Could you check a few things on this model? Use its own coordinates, in mm. A direction names the side the tool comes from. Give positions to 0.01 mm unless a question says otherwise; leave off trailing zeros. Loops run counter-clockwise (first coordinate to the right, second up) from the corner with the lowest first, then second, coordinate; pieces in that order, holes last. Notation, with made-up numbers: M -20,43 L 21,43 A26 ccw 21,75 Z; hole C -12,-17 d7. An arc over 180 degrees is marked long. Return JSON: item names as keys, results as strings. Group by question number.
1. If we section it at A-A (y = -23): Write out the boundary of the cut face in (x, z), plus the area to 3 significant figures.
2. Please list where these lines run through material, in increasing order: line 1 (Y direction, x = -20.5, z = 41); line 2 (X direction, y = -4, z = 31.5); line 3 (X direction, y = -6, z = 130).
3. If we section it at C-C (x = 125.5): Write out the boundary of the cut face in (y, z).
4. If we mould it in two halves opening along Z, with no side actions, what happens to faces 4 (the cylindrical face through (86.45, -3.13, 20.73)), 5 (the flat face through (41, -6.35, 53)), 6 (the cylindrical face through (-39.79, -3.22, 1.59))? For each: +Z half, -Z half, draft (parallel to the pull), parting line (faces both ways), or undercut.
5. For faces 1 (the flat face through (162.27, -18.87, 120.88)), 2 (the cylindrical face through (39.885, -3.219, 1.509)), 3 (the flat face through (41, 0, 53)), which set-ups out of +Z, -Z, +X, -X, +Y, -Y let a thin tool reach every point of the face, with its end or its side?
6. If we section it at B-B (z = 80): Write out the boundary of the cut face in (x, y), plus the area to 3 significant figures.
7. For pin 1 (8 mm diameter, centred on y = -15.5, z = 98, fed in from -X); pin 2 (12 mm diameter, centred on x = -55.99, z = 55.99, fed in from -Y); pin 3 (8 mm diameter, centred on x = 127.5, y = -13.5, fed in from +Z), each with a flat end and sliding along its axis, tell me the tip position at first contact or that it passes through.
8. If we section it at D-D (y = -9.5): Write out the boundary of the cut face in (x, z), plus the area to 3 significant figures.
```python
from build123d import *

# Parameters (mm, degrees)
F1_DEPTH = 6.35
F3_D     = 10.3124
F5_DEPTH = 25.4
F7_D     = 14
F8_R     = 12.7
F9_R     = 5.08
F10_R    = 6.35


# Not quite as in the source:
# - a feature names something its author has since deleted; it is built from what else it names


with BuildPart() as f1:
    # F0 (on Front) → F1 (new body)
    with BuildSketch(Plane.XZ):
        with BuildLine():
            Line((38.1, 0), (88.9, 0))
            ThreePointArc((88.9, 0), (85.8708059571, 23.0090131096), (76.9896583964, 44.45))
            Line((76.9896583964, 44.45), (179.5459910838, 103.6609262841))
            Line((179.5459910838, 103.6609262841), (160.4959910838, 136.6564941683))
            Line((160.4959910838, 136.6564941683), (50.5107648032, 73.1564941683))
            ThreePointArc((50.5107648032, 73.1564941683), (-41.3086129578, 78.7198100576), (-88.9, 0))
            Line((-88.9, 0), (-38.1, 0))
            ThreePointArc((-38.1, 0), (0, 38.1), (38.1, 0))
        make_face()
    extrude(amount=F1_DEPTH)

    # F3 (through all)
    with Locations(Plane.XZ.offset(6.35)):
        with Locations((-55.9918969149, 55.9918969149), (55.9918969149, 55.9918969149)):
            Hole(F3_D / 2)

    # F4 (on face) → F5 (join)
    with BuildSketch(Plane.XZ.offset(6.35)):
        Polygon((160.4959910838, 136.6564941683), (154.9967297697, 133.4814941683), (174.0467297697, 100.4859262841), (179.5459910838, 103.6609262841), align=None)
    extrude(amount=F5_DEPTH)

    # F7 (through all)
    with Locations(Plane(origin=(174.0467297697, 0, 100.4859262841), x_dir=(0, -1, 0), z_dir=(-0.8660254038, 0, -0.5))):
        with Locations((19.05, 12.7)):
            Hole(F7_D / 2)

    # F8
    f8_edges = [f1.edges().sort_by_distance(p)[0] for p in [
        (50.510765, -3.175, 73.156494),
        (76.989658, -3.175, 44.45),
    ]]
    fillet(f8_edges, radius=F8_R)

    # F9
    f9_edges = [f1.edges().sort_by_distance(p)[0] for p in [
        (170.020991, 0, 120.15871),
    ]]
    fillet(f9_edges, radius=F9_R)

    # F10
    f10_edges = [f1.edges().sort_by_distance(p)[0] for p in [
        (88.9, -3.175, 0),
        (38.1, -3.175, 0),
        (-38.1, -3.175, 0),
        (-88.9, -3.175, 0),
    ]]
    fillet(f10_edges, radius=F10_R)


solid = f1.part
```
Answer:
{
 "1": {"outline": "M 155,133.48 L 164.81,116.49 L 170.31,119.66 L 160.5,136.66 Z; M 170.59,106.48 L 174.05,100.49 L 179.55,103.66 L 176.09,109.65 Z", "area": "169 mm²"},
 "2": {"line 1": "y = -6.35 to 0", "line 2": "x = -83.13 to -21.43, 21.43 to 83.13", "line 3": "x = 148.97 to 164.34"},
 "3": {"outline": "M -6.35,72.46 L 0,72.46 L 0,116.45 L -6.35,116.45 Z"},
 "4": {"face 4": "undercut", "face 5": "draft", "face 6": "-Z half"},
 "5": {"face 1": "-Z, -X, -Y", "face 2": "-Z, +Y, -Y", "face 3": "+Z, -Z, +X, -X, +Y"},
 "6": {"outline": "M -38.77,-6.35 L 38.77,-6.35 L 38.77,0 L -38.77,0 Z; M 62.36,-6.35 L 138.56,-6.35 L 138.56,0 L 62.36,0 Z", "area": "976 mm²"},
 "7": {"pin 1": "stops at x = 173.17", "pin 2": "stops at y = -6.35", "pin 3": "passes through"},
 "8": {"outline": "M 155,133.48 L 174.05,100.49 L 179.55,103.66 L 160.5,136.66 Z", "area": "242 mm²"}
}
